For this review, take the finished solid that the model builds, in its own axes (mm). A direction names the side the tool comes from. Round coordinates to 2 decimals unless told otherwise and drop trailing zeros. Order: outer loops, then holes, each group sorted by start corner. A loop starts at its lowest first (then second) coordinate and runs counter-clockwise, first axis right, second up. Notation, with made-up numbers: (50.25, -8.5) - (79.25, -8.5) arc R10 cw to (79.25, -3.5) - close; hole circle Ø10 at (39.25, 37.25). An arc over 180 degrees is marked (long way). One line per item, written item: value.
```python
from build123d import *

# Parameters (mm, degrees)
BOSS_EXTRUDE1_DEPTH = 44
SKETCH5_R           = 7
CUT_EXTRUDE1_DEPTH  = 171.828393793
CHAMFER1_SIZE       = 7
CHAMFER2_SIZE       = 7
CHAMFER3_SIZE       = 5
SKETCH8_R           = 6.128605104
CUT_EXTRUDE2_DEPTH  = 171.828393793
SKETCH9_W           = 34
SKETCH9_H           = 19
CUT_EXTRUDE3_DEPTH  = 168.605610181
CUT_EXTRUDE4_START  = -12
CUT_EXTRUDE4_DEPTH  = 24


with BuildPart() as part:
    # Sketch4 → Boss-Extrude1 (new body)
    with BuildSketch(Plane.XY):
        with BuildLine():
            Line((-153.475211562, 21.759357812), (-153.475211562, 53.759357812))
            Line((-153.475211562, 53.759357812), (-139.475211562, 53.759357812))
            Line((-139.475211562, 53.759357812), (-117.113830726, 49.816443045))
            ThreePointArc((-117.113830726, 49.816443045), (-104.914112856, 51.741401954), (-96.475211562, 60.759357812))
            Line((-96.475211562, 60.759357812), (-67.475211562, 60.759357812))
            Line((-67.475211562, 60.759357812), (-67.475211562, 36.759357812))
            Line((-67.475211562, 36.759357812), (-96.475211562, 2.759357812))
            Line((-96.475211562, 2.759357812), (-102.178231509, 2.759357812))
            ThreePointArc((-102.178231509, 2.759357812), (-106.617203706, 9.643685751), (-108.954033909, 17.49465193))
            ThreePointArc((-108.954033909, 17.49465193), (-110.63443687, 20.545944044), (-113.899672651, 21.759357812))
            Line((-113.899672651, 21.759357812), (-153.475211562, 21.759357812))
        make_face()
    extrude(amount=BOSS_EXTRUDE1_DEPTH)

    # Sketch5 → Cut-Extrude1 (cut, through all)
    with BuildSketch(Plane.XY):
        with Locations((-139.475211562, 35.759357812)):
            Circle(SKETCH5_R)
    extrude(amount=CUT_EXTRUDE1_DEPTH, mode=Mode.SUBTRACT)

    # Chamfer1
    chamfer1_edges = [part.edges().sort_by_distance(p)[0] for p in [
        (-153.475211562, 53.759357812, 22),
    ]]
    chamfer(chamfer1_edges, length=CHAMFER1_SIZE)

    # Chamfer2
    chamfer2_edges = [part.edges().sort_by_distance(p)[0] for p in [
        (-153.475211562, 21.759357812, 22),
    ]]
    chamfer(chamfer2_edges, length=CHAMFER2_SIZE)

    # Chamfer3
    chamfer3_edges = [part.edges().sort_by_distance(p)[0] for p in [
        (-67.475211562, 60.759357812, 22),
    ]]
    chamfer(chamfer3_edges, length=CHAMFER3_SIZE)

    # Sketch8 → Cut-Extrude2 (cut, through all)
    with BuildSketch(Plane.XY.offset(44)):
        with Locations((-81.475211562, 46.759357812)):
            Circle(SKETCH8_R)
    extrude(amount=-CUT_EXTRUDE2_DEPTH, mode=Mode.SUBTRACT)

    # Sketch9 → Cut-Extrude3 (cut, through all)
    with BuildSketch(Plane(origin=(0, 53.759357812, 0), x_dir=(1, 0, 0), z_dir=(0, 1, 0))):
        with Locations((-136.475211562, -34.5)):
            Rectangle(SKETCH9_W, SKETCH9_H)
    extrude(amount=-CUT_EXTRUDE3_DEPTH, mode=Mode.SUBTRACT)

    # Sketch10 → Cut-Extrude4 (cut)
    with BuildSketch(Plane(origin=(0, 0, 0), x_dir=(-1, 0, 0), z_dir=(0, 0, -1)).offset(CUT_EXTRUDE4_START)):
        with BuildLine():
            Line((77.71050568, 24.759357812), (67.475211562, 36.759357812))
            Line((67.475211562, 36.759357812), (67.475211562, 55.759357812))
            Line((67.475211562, 55.759357812), (72.475211562, 60.759357812))
            Line((72.475211562, 60.759357812), (96.475211562, 60.759357812))
            ThreePointArc((96.475211562, 60.759357812), (100.453967219, 55.018691433), (106.238275013, 51.103652429))
            ThreePointArc((106.238275013, 51.103652429), (95.290948579, 34.340063041), (77.71050568, 24.759357812))
        make_face()
    extrude(amount=-CUT_EXTRUDE4_DEPTH, mode=Mode.SUBTRACT)


solid = part.part
```
Item 1: Take a section at A-A (z = 39). Write out the cut boundary in (x, y), plus the area to 3 significant figures.
Returned:
outline: (-119.48, 21.76) - (-113.9, 21.76) arc R5 cw to (-108.95, 17.49) arc R29 ccw to (-102.18, 2.76) - (-96.48, 2.76) - (-67.48, 36.76) - (-67.48, 55.76) - (-72.48, 60.76) - (-96.48, 60.76) arc R19 cw to (-117.11, 49.82) - (-119.48, 50.23) - close; hole circle Ø12.26 at (-81.48, 46.76)
area: 1,960 mm^2
Item 2: Take a section at B-B (y = 45). Write out the cut boundary in (x, z).
Returned:
outline: (-153.48, 0) - (-87.35, 0) - (-87.35, 12) - (-103.56, 12) - (-103.56, 36) - (-87.35, 36) - (-87.35, 44) - (-119.48, 44) - (-119.48, 25) - (-153.48, 25) - close; (-75.6, 0) - (-67.48, 0) - (-67.48, 12) - (-75.6, 12) - close; (-75.6, 36) - (-67.48, 36) - (-67.48, 44) - (-75.6, 44) - close
Item 3: The part is to be moulded in two halves that separate along Y. For faces 5 (the cylindrical face through (-135.71, 41.66, 12.32)), 6 (the flat face through (-69.94, 58.224, 5.916)), 7 (the flat face through (-93, 39, 44)), say which applies: +Y half, -Y half, draft (parallel to the pull), parting line (faces both ways), or undercut.
Returned:
face 5: undercut
face 6: +Y half
face 7: draft
Item 4: For P1, Ø1.5, axis at y = 14.5, z = 13.5, coming from the +X side; P2, Ø5, axis at x = -86.5, z = 29, coming from the -Y side; P3, Ø3, axis at x = -120.5, z = 22.5, coming from the +Y side, all flat-tipped, find the tip position at first contact; note any pin that passes through.
Returned:
P1: x = -85.82
P2: y = 11.52
P3: y = 50.68
Item 5: Wall thickness on line 1 (Z direction, x = -99.5, y = 50); line 2 (Z direction, x = -123, y = 27); line 3 (X direction, y = 45, z = 3): over which ranges is each line inside the solid? List them lowest first.
Returned:
line 1: 0 to 12, 36 to 44
line 2: 0 to 25
line 3: -153.48 to -87.35, -75.6 to -67.48
Item 6: Take a section at C-C (x = -79.5). Write out the cut boundary in (y, z), plus the area to 3 significant figures.
Returned:
outline: (22.66, 0) - (40.96, 0) - (40.96, 12) - (25.26, 12) - (25.26, 36) - (40.96, 36) - (40.96, 44) - (22.66, 44) - close; (52.56, 0) - (60.76, 0) - (60.76, 12) - (52.56, 12) - close; (52.56, 36) - (60.76, 36) - (60.76, 44) - (52.56, 44) - close
area: 592 mm^2
Item 7: Take a section at D-D (z = 10). Write out the cut boundary in (x, y), plus the area to 3 significant figures.
Returned:
outline: (-153.48, 28.76) - (-146.48, 21.76) - (-113.9, 21.76) arc R5 cw to (-108.95, 17.49) arc R29 ccw to (-102.18, 2.76) - (-96.48, 2.76) - (-67.48, 36.76) - (-67.48, 55.76) - (-72.48, 60.76) - (-96.48, 60.76) arc R19 cw to (-117.11, 49.82) - (-139.48, 53.76) - (-146.48, 53.76) - (-153.48, 46.76) - close; hole circle Ø14 at (-139.48, 35.76); hole circle Ø12.26 at (-81.48, 46.76)
area: 2,810 mm^2
Item 8: Machinability: for faces 1 (the flat face through (-119.475, 36, 35)), 2 (the flat face through (-87, 43, 36)), 3 (the flat face through (-143, 53.759, 12)), 4 (the flat face through (-128.451, 51.816, 11.914)), which of the approach directions +Z, -Z, +X, -X, +Y, -Y give a long, thin tool a straight path to every point of the face, cutting with its end or side? Answer none if there is none.
Returned:
face 1: +Z, -X, +Y, -Y
face 2: +X, +Y
face 3: +Z, -Z, -X, +Y
face 4: +Z, -Z, +Y
